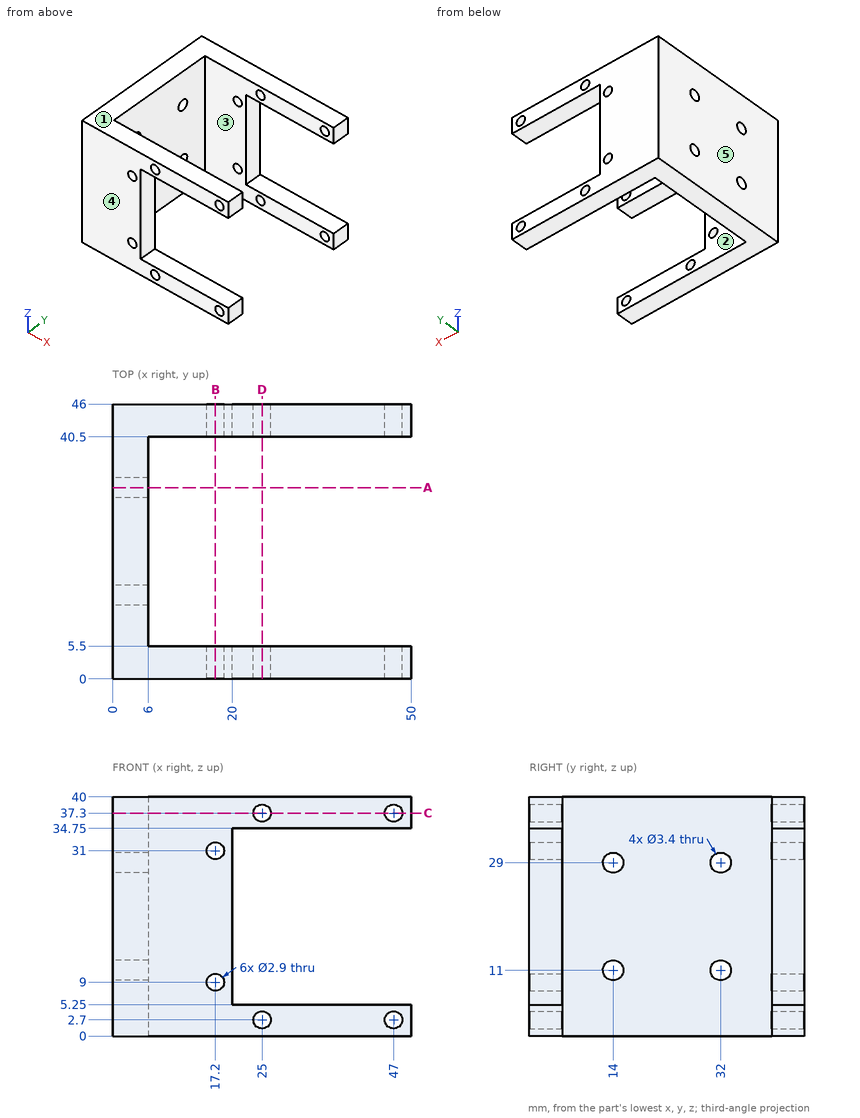
Study the drawing (mm; zero at the part's minimum x, y, z) and answer. A direction names the side the tool comes from. Round coordinates to 2 decimals unless told otherwise and drop trailing zeros. Order: outer loops, then holes, each group sorted by start corner. A loop starts at its lowest first (then second) coordinate and runs counter-clockwise, first axis right, second up. Notation, with made-up numbers: (31, 89.25) -> (68, 89.25) arc R18 cw to (68, 111.25) -> close; hole circle Ø4 at (4.5, 38). An arc over 180 degrees is marked (long way). Answer as CSV lines item,"result". Start each with the question number.
(1) Find the intervals of material crossed by probe 1 along Z at (x, y) = (17, 2); probe 2 along Z at (x, y) = (4.2, 32); probe 3 along Y at (x, z) = (44.5, 2), in increasing order. Write a range as from..to.
(2) The part is cut by section B-B (x = 17.2). Determine the outline of the cut face in (y, z), then the cut area to 3 significant figures.
(3) The part is cut by section D-D (x = 25). Count the separate pieces of the cut face and the enclosed holes in it, then the cut area to 3 significant figures.
(4) The part is cut by section A-A (y = 32). Determine the outline of the cut face in (x, z).
(5) The part is cut by section C-C (z = 37.3). Determine the outline of the cut face in (x, y).
(6) Flat-ended cylindrical pins translate along their axes: pin 1 Ø8 at (y, z) = (20.5, 28) entering from +X; pin 2 Ø3 at (y, z) = (44, 13) entering from +X. Find the tip coordinate at first contact, or state that the pin passes through.
(7) A tool of negligible diameter and unlimited length cuts with its end or side. For the marked faces 1 and 2, from which of +Z, -Z, +X, -X, +Y, -Y can it reach the whole face along a straight path? Write none if from no direction.
(8) For a pull along Y with two mould halves and no side action, classify the marked faces 3, 4 and 5 as +Y half, -Y half, draft (parallel to the pull), parting line (faces both ways), or undercut.
Evaluation:
1,probe 1,"0..7.56, 10.44..29.56, 32.44..40"
1,probe 2,"0..9.3, 12.7..27.3, 30.7..40"
1,probe 3,"0..5.5, 40.5..46"
2,outline,"(0, 0) -> (5.5, 0) -> (5.5, 7.55) -> (0, 7.55) -> close; (0, 10.45) -> (5.5, 10.45) -> (5.5, 29.55) -> (0, 29.55) -> close; (0, 32.45) -> (5.5, 32.45) -> (5.5, 40) -> (0, 40) -> close; (40.5, 0) -> (46, 0) -> (46, 7.55) -> (40.5, 7.55) -> close; (40.5, 10.45) -> (46, 10.45) -> (46, 29.55) -> (40.5, 29.55) -> close; (40.5, 32.45) -> (46, 32.45) -> (46, 40) -> (40.5, 40) -> close"
2,area,"376 mm²"
3,separate pieces,"8"
3,enclosed holes,"0"
3,area,"51.7 mm²"
4,outline,"(0, 0) -> (6, 0) -> (6, 9.3) -> (0, 9.3) -> close; (0, 12.7) -> (6, 12.7) -> (6, 27.3) -> (0, 27.3) -> close; (0, 30.7) -> (6, 30.7) -> (6, 40) -> (0, 40) -> close"
5,outline,"(0, 0) -> (23.55, 0) -> (23.55, 5.5) -> (6, 5.5) -> (6, 40.5) -> (23.55, 40.5) -> (23.55, 46) -> (0, 46) -> close; (26.45, 0) -> (45.55, 0) -> (45.55, 5.5) -> (26.45, 5.5) -> close; (26.45, 40.5) -> (45.55, 40.5) -> (45.55, 46) -> (26.45, 46) -> close; (48.45, 0) -> (50, 0) -> (50, 5.5) -> (48.45, 5.5) -> close; (48.45, 40.5) -> (50, 40.5) -> (50, 46) -> (48.45, 46) -> close"
6,pin 1,"x = 6"
6,pin 2,"x = 20"
7,face 1,"+Z, +X, -X, +Y, -Y"
7,face 2,"+Z, -Z, +X"
8,face 3,"undercut"
8,face 4,"-Y half"
8,face 5,"draft"
